Geometry check sheet. Reference: the model listing, model coordinates, mm. Face numbers are marked on the shaded views. A direction names the side the tool comes from. Give positions to 0.01 mm unless a question says otherwise; leave off trailing zeros. Write each loop counter-clockwise with the first axis right and the second up, starting at its lowest first coordinate (ties: lowest second). Pieces come first, ordered by that corner, then holes. Notation, with made-up numbers: M 83,29.25 L 122,29.25 A18 cw 122,41.25 Z; hole C 70,-4.5 d7. An arc over 180 degrees is marked long. One line per item, written item: value. Start each with the question number.
1. Tool access check on the marked faces 4, 5 and 6. Record the directions out of +Z, -Z, +X, -X, +Y, -Y that give a thin tool (end or side, any length) a straight path to the whole face; none if there is none.
2. Cross-section at A-A on x = 6. Record the cut outline in (y, z).
3. Scan lines: line 1 (X direction, y = 3, z = -65); line 2 (Z direction, x = 35.5, y = 17); line 3 (Z direction, x = 65, y = 3.45). Record each from-to range of solid material in increasing order.
4. Gauge pin test, flat ends, axial feed: pin 1 (12 mm diameter, centred on x = 43, y = 20, fed in from +Z); pin 2 (5 mm diameter, centred on y = 22.5, z = -36, fed in from -X); pin 3 (2 mm diameter, centred on x = 42.5, y = 22, fed in from -Z); pin 4 (1.8 mm diameter, centred on x = 65, z = -65, fed in from +Y). Record the tip position at first contact, or that the pin passes through.
5. Release check for a two-part mould opening along Z. For the marked faces 1, 2 and 3 record: pulls with the +Z half, pulls with the -Z half, needs draft (parallel to the pull), parting line crosses it, or undercut.
6. Cross-section at B-B on z = -6. Record the cut outline in (x, y).
7. Cross-section at C-C on y = 8.5. Record the cut outline in (x, z), then the cut area to 3 significant figures.
8. Cross-section at D-D on x = 59.5. Record the cut outline in (y, z).
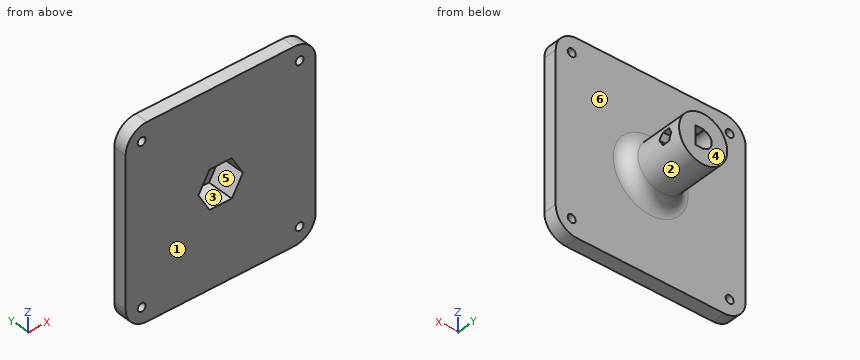
from build123d import *

# Parameters (mm, degrees)
SKETCH1_W               = 71
SKETCH1_H               = 71
BOSS_EXTRUDE1_DEPTH     = 5
SKETCH2_R               = 9
BOSS_EXTRUDE2_DEPTH     = 23
FILLET1_R               = 5
CUT_EXTRUDE1_DEPTH      = 46
FILLET2_R               = 8
SKETCH4_R               = 1.5
CUT_EXTRUDE2_DEPTH      = 6
CUT_EXTRUDE3_DEPTH      = 10
CUT_EXTRUDE4_DEPTH      = 2.5
CUT_EXTRUDE4_DEPTH_BACK = 3.35
FILLET3_R               = 0.5
CUT_EXTRUDE9_DEPTH      = 30.95
SKETCH11_W              = 3.248200577
SKETCH11_H              = 7
CUT_EXTRUDE10_DEPTH     = 5


with BuildPart() as part:
    # Sketch1 → Boss-Extrude1 (new body)
    with BuildSketch(Plane(origin=(0, 0, 0), x_dir=(1, 0, 0), z_dir=(0, 1, 0))):
        with Locations((35.5, 35.5)):
            Rectangle(SKETCH1_W, SKETCH1_H)
    extrude(amount=BOSS_EXTRUDE1_DEPTH)

    # Sketch2 → Boss-Extrude2 (add)
    with BuildSketch(Plane(origin=(0, 5, 0), x_dir=(1, 0, 0), z_dir=(0, 1, 0))):
        with Locations((35.5, 35.5)):
            Circle(SKETCH2_R)
    extrude(amount=BOSS_EXTRUDE2_DEPTH)

    # Fillet1
    fillet1_edges = [part.edges().sort_by_distance(p)[0] for p in [
        (26.5, 5, -35.5),
    ]]
    fillet(fillet1_edges, radius=FILLET1_R)

    # Sketch3 → Cut-Extrude1 (cut)
    with BuildSketch(Plane(origin=(0, 28, 0), x_dir=(1, 0, 0), z_dir=(0, 1, 0))):
        with BuildLine():
            Line((37.7, 33.176209992), (37.7, 37.823790008))
            ThreePointArc((37.7, 37.823790008), (32.3, 35.5), (37.7, 33.176209992))
        make_face()
    extrude(amount=-CUT_EXTRUDE1_DEPTH, mode=Mode.SUBTRACT)

    # Fillet2
    fillet2_edges = [part.edges().sort_by_distance(p)[0] for p in [
        (0, 2.5, -71),
        (71, 2.5, -71),
        (71, 2.5, 0),
        (0, 2.5, 0),
    ]]
    fillet(fillet2_edges, radius=FILLET2_R)

    # Sketch4 → Cut-Extrude2 (cut, through all)
    with BuildSketch(Plane(origin=(0, 5, 0), x_dir=(1, 0, 0), z_dir=(0, 1, 0))):
        with Locations((65, 65)):
            Circle(SKETCH4_R)
        with Locations((65, 6)):
            Circle(SKETCH4_R)
        with Locations((6, 6)):
            Circle(SKETCH4_R)
        with Locations((6, 65)):
            Circle(SKETCH4_R)
    extrude(amount=-CUT_EXTRUDE2_DEPTH, mode=Mode.SUBTRACT)

    # Sketch5 → Cut-Extrude3 (cut)
    with BuildSketch(Plane(origin=(0, 0, 0), x_dir=(-1, 0, 0), z_dir=(0, -1, 0))):
        Polygon((-43.813843876, 35.5), (-39.656921938, 28.3), (-31.343078062, 28.3), (-27.186156124, 35.5), (-31.343078062, 42.7), (-39.656921938, 42.7), align=None)
    extrude(amount=-CUT_EXTRUDE3_DEPTH, mode=Mode.SUBTRACT)

    # Sketch6 → Cut-Extrude4 (cut, two sides)
    with BuildSketch(Plane.ZY.offset(-37.7)) as cut_extrude4_sk:
        Polygon((-35.456209992, 26.041451884), (-38.956209992, 24.020725942), (-38.956209992, 19.979274058), (-35.456209992, 17.958548116), (-31.956209992, 19.979274058), (-31.956209992, 24.020725942), align=None)
    extrude(amount=CUT_EXTRUDE4_DEPTH, mode=Mode.SUBTRACT)
    extrude(cut_extrude4_sk.sketch, amount=-CUT_EXTRUDE4_DEPTH_BACK, mode=Mode.SUBTRACT)

    # Fillet3
    fillet3_edges = [part.edges().sort_by_distance(p)[0] for p in [
        (41.05, 25.031088913, -33.706209992),
        (41.05, 25.031088913, -37.206209992),
        (41.05, 22, -38.956209992),
        (41.05, 18.968911087, -37.206209992),
        (41.05, 18.968911087, -33.706209992),
        (41.05, 22, -31.956209992),
    ]]
    fillet(fillet3_edges, radius=FILLET3_R)

    # Sketch10 → Cut-Extrude9 (cut, through all)
    with BuildSketch(Plane.ZY.offset(-41.05)):
        Polygon((-35.456209992, 24.629291376), (-37.756209992, 23.301385757), (-37.756209992, 20.645574519), (-35.456209992, 19.3176689), (-33.156209992, 20.645574519), (-33.156209992, 23.301385757), align=None)
    extrude(amount=-CUT_EXTRUDE9_DEPTH, mode=Mode.SUBTRACT)

    # Sketch11 → Cut-Extrude10 (cut)
    with BuildSketch(Plane(origin=(0, 28, 0), x_dir=(1, 0, 0), z_dir=(0, 1, 0))):
        with Locations((36.824100289, 35.456209992)):
            Rectangle(SKETCH11_W, SKETCH11_H)
    extrude(amount=-CUT_EXTRUDE10_DEPTH, mode=Mode.SUBTRACT)


solid = part.part
Report:
1. face 4: +Z, -Z, +X, -X, +Y
1. face 5: -Y
1. face 6: +Y
2. outline: M 0,-70.75 L 5,-70.75 L 5,-66.5 L 0,-66.5 Z; M 0,-63.5 L 5,-63.5 L 5,-7.5 L 0,-7.5 Z; M 0,-4.5 L 5,-4.5 L 5,-0.25 L 0,-0.25 Z
3. line 1: x = 0.25 to 4.5, 7.5 to 63.5, 66.5 to 70.75
3. line 2: z = -44.5 to -38.7, -32.3 to -26.5
3. line 3: z = -70.75 to -66.5, -63.5 to -7.5, -4.5 to -0.25
4. pin 1: stops at z = -26.63
4. pin 2: stops at x = 26.5
4. pin 3: stops at z = -42.21
4. pin 4: passes through
5. face 1: needs draft
5. face 2: parting line crosses it
5. face 3: undercut
6. outline: M 0.25,0 L 4.5,0 L 4.5,5 L 0.25,5 Z; M 7.5,0 L 63.5,0 L 63.5,5 L 7.5,5 Z; M 66.5,0 L 70.75,0 L 70.75,5 L 66.5,5 Z
7. outline: C 35.5,-35.5 d18.46; hole M 27.19,-35.5 L 31.34,-42.7 L 39.66,-42.7 L 43.81,-35.5 L 39.66,-28.3 L 31.34,-28.3 Z
7. area: 88.1 mm^2
8. outline: M 0,-71 L 5,-71 L 5,0 L 0,0 Z
